Verification items for the finished model (mm, model axes). A direction names the side the tool comes from. Coordinates: 2 decimals unless noted, no trailing zeros. Order: outer loops, then holes, each group sorted by start corner. A loop starts at its lowest first (then second) coordinate and runs counter-clockwise, first axis right, second up. Notation, with made-up numbers: M 77,-30.75 L 130,-30.75 A18 ccw 130,-16.75 Z; hole C 44,80.5 d10. An arc over 180 degrees is marked long. Return JSON: item names as keys, results as strings.
```python
from build123d import *

# Parameters (mm, degrees)
SKETCH1_W                = 90.23
SKETCH1_H                = 24
BOSS_EXTRUDE1_DEPTH      = 20
FILLET1_R                = 20
SKETCH2_W                = 6.48
SKETCH2_H                = 19.05
CUT_EXTRUDE1_DEPTH       = 0.64
M2_CLEARANCE_HOLE1_D     = 2.6
M2_CLEARANCE_HOLE1_DEPTH = 2
M2_CLEARANCE_HOLE1_TIP   = 0.781118805
SKETCH5_R                = 15.08
CUT_EXTRUDE2_DEPTH       = 5.56
SKETCH6_R                = 11.905
CUT_EXTRUDE3_DEPTH       = 11.1


with BuildPart() as part:
    # Sketch1 → Boss-Extrude1 (new body)
    with BuildSketch(Plane(origin=(0, 0, 0), x_dir=(1, 0, 0), z_dir=(0, 1, 0))):
        Rectangle(SKETCH1_W, SKETCH1_H)
    extrude(amount=BOSS_EXTRUDE1_DEPTH)

    # Fillet1
    fillet1_edges = [part.edges().sort_by_distance(p)[0] for p in [
        (45.115, 20, 0),
        (-45.115, 20, 0),
    ]]
    fillet(fillet1_edges, radius=FILLET1_R - 0.0001)  # a hair under: the kernel refuses the full size

    # Sketch2 → Cut-Extrude1 (cut)
    with BuildSketch(Plane.XZ):
        with Locations((41.875, 0)):
            Rectangle(SKETCH2_W, SKETCH2_H)
    extrude(amount=-CUT_EXTRUDE1_DEPTH, mode=Mode.SUBTRACT)

    # M2 Clearance Hole1
    with Locations(Plane(origin=(0, 0.64, 0), x_dir=(-1, 0, 0), z_dir=(0, -1, 0))):
        with Locations((-41.875, 5.565), (-41.875, -5.565)):
            Hole(M2_CLEARANCE_HOLE1_D / 2, depth=M2_CLEARANCE_HOLE1_DEPTH)
            with Locations((0, 0, -(M2_CLEARANCE_HOLE1_DEPTH + M2_CLEARANCE_HOLE1_TIP / 2))):  # 118° drill point
                Cone(0, M2_CLEARANCE_HOLE1_D / 2, M2_CLEARANCE_HOLE1_TIP, mode=Mode.SUBTRACT)

    # Sketch5 → Cut-Extrude2 (cut)
    with BuildSketch(Plane.XZ):
        Circle(SKETCH5_R)
    extrude(amount=-CUT_EXTRUDE2_DEPTH, mode=Mode.SUBTRACT)

    # Sketch6 → Cut-Extrude3 (cut)
    with BuildSketch(Plane.XZ.offset(-5.56)):
        with Locations(Location((0, 0, 0), (0, 0, 270))):
            Circle(SKETCH6_R)
    extrude(amount=-CUT_EXTRUDE3_DEPTH, mode=Mode.SUBTRACT)


solid = part.part
```
Q1. Material ranges on line 1 along Y through (x, z) = (-3, 7.75); line 2 along X through (y, z) = (5, -2); line 3 along Z through (x, y) = (2.5, 13.25), recorded low to high.
Values:
{"line 1": "16.66 to 20", "line 2": "-44.48 to -14.95, 14.95 to 44.48", "line 3": "-12 to -11.64, 11.64 to 12"}
Q2. Cross-section at D-D, the plane y = 6.75. Record the boundary of the cut face in (x, z) (3 decimals).
Values:
{"outline": "M -43.942,-12 L 43.942,-12 L 43.942,12 L -43.942,12 Z; hole C 0,0 d23.81"}
Q3. Cross-section at A-A, the plane x = 0. Record the boundary of the cut face in (y, z) (3 decimals).
Values:
{"outline": "M 5.56,-12 L 20,-12 L 20,12 L 5.56,12 L 5.56,11.905 L 16.66,11.905 L 16.66,-11.905 L 5.56,-11.905 Z"}
Q4. Tool access check on faces 4 (the face through (40.576, 1.654, -5.622)), 5 (the face through (0, 20, 0)), 6 (the face through (42, 0.64, 0)). Record the directions out of +Z, -Z, +X, -X, +Y, -Y that give a thin tool (end or side, any length) a straight path to the whole face; none if there is none.
Values:
{"face 4": "-Y", "face 5": "+Z, -Z, +X, -X, +Y", "face 6": "+X, -Y"}
Q5. Cross-section at C-C, the plane y = 14.5. Record the boundary of the cut face in (x, z) (3 decimals).
Values:
{"outline": "M -38.89,-12 L 38.89,-12 L 38.89,12 L -38.89,12 Z; hole C 0,0 d23.81"}
Q6. Draft check along X on faces 1 (the face through (-27, 0, 0)), 2 (the face through (-15.08, 2.74, 0.19)), 3 (the face through (-39.4, 14, -0.2)). Enter one of: pulls with the +X half, pulls with the -X half, needs draft (parallel to the pull), parting line crosses it, or undercut.
Values:
{"face 1": "needs draft", "face 2": "undercut", "face 3": "pulls with the -X half"}
Q7. Go/stop test with flat-tipped pins: pin 1 (7 mm diameter, centred on x = -0.5, z = 2.5, fed in from -Y); pin 2 (2 mm diameter, centred on y = 7, z = -9.5, fed in from -X); pin 3 (1.6 mm diameter, centred on x = 41.875, z = -5.565, fed in from +Y). Record where each tip stops, or that it passes through.
Values:
{"pin 1": "y = 16.66", "pin 2": "x = -44.19", "pin 3": "y = 12.05"}
